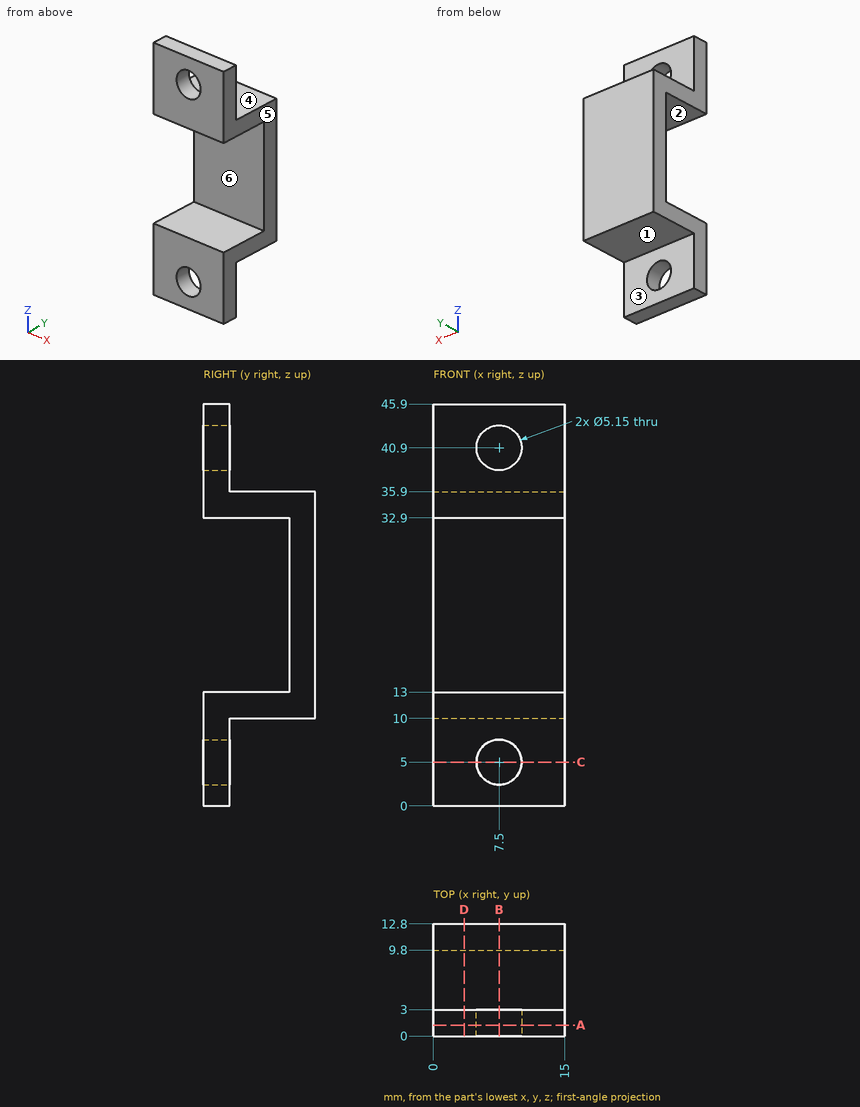
Job drawing, mm, ordinate dimensions from the low corner. One solid piece. A direction names the side the tool comes from. Round coordinates to 2 decimals unless told otherwise and drop trailing zeros. Loops run counter-clockwise (first coordinate to the right, second up) from the corner with the lowest first, then second, coordinate; pieces in that order, holes last. Notation, with made-up numbers: M -11.5,68 L 5.5,68 A34 cw 5.5,106 Z; hole C 31,83 d6. An arc over 180 degrees is marked long. One line per question, with ' | ' between items. Start each with the question number.
Item 1: Wall check: line 1 (Z direction, x = 7.5, y = 1.7) (3 decimals); line 2 (Z direction, x = 6, y = 7.5); line 3 (Z direction, x = 3.75, y = 0.5). Give the ranges that are in metal, low to high.
Item 2: Cut at C-C, the plane z = 5. Write the cut outline in (x, y) (3 decimals).
Item 3: Cut at B-B, the plane x = 7.5. Write the cut outline in (y, z) (3 decimals), plus the area to 3 significant figures.
Item 4: Cut at A-A, the plane y = 1.25. Write the cut outline in (x, z) (3 decimals), plus the area to 3 significant figures.
Item 5: Pin check, flat tips, straight feed: pin 1 Ø5 at (x, z) = (8.5, 39.5) entering from +Y; pin 2 Ø2 at (x, y) = (10.5, 9.5) entering from -Z; pin 3 Ø3 at (x, y) = (7, 6) entering from +Z. Stop position of each tip, or through.
Item 6: Cut at D-D, the plane x = 3.5. Write the cut outline in (y, z), plus the area to 4 significant figures.
Item 7: Two-plate mould, pull along Z, no slides. Class the marked faces 1, 2 and 3: pulls with the +Z half, pulls with the -Z half, needs draft (parallel to the pull), parting line crosses it, or undercut.
Item 8: Which spindle directions (+Z, -Z, +X, -X, +Y, -Y) get a long thin tool onto all of the face, cutting with end or side? Do the marked faces 4, 5 and 6. Say none if no direction does.
Responses:
1) line 1: z = 0 to 2.425, 7.575 to 13, 32.9 to 38.325, 43.475 to 45.9 | line 2: z = 10 to 13, 32.9 to 35.9 | line 3: z = 0 to 13, 32.9 to 45.9
2) outline: M 0,0 L 4.925,0 L 4.925,3 L 0,3 Z; M 10.075,0 L 15,0 L 15,3 L 10.075,3 Z
3) outline: M 0,0 L 3,0 L 3,2.425 L 0,2.425 Z; M 0,7.575 L 3,7.575 L 3,10 L 12.8,10 L 12.8,35.9 L 3,35.9 L 3,38.325 L 0,38.325 L 0,32.9 L 9.8,32.9 L 9.8,13 L 0,13 Z; M 0,43.475 L 3,43.475 L 3,45.9 L 0,45.9 Z | area: 166 mm²
4) outline: M 0,0 L 15,0 L 15,13 L 0,13 Z; M 0,32.9 L 15,32.9 L 15,45.9 L 0,45.9 Z; hole C 7.5,5 d5.15; hole C 7.5,40.9 d5.15 | area: 348 mm²
5) pin 1: stops at y = 3 | pin 2: stops at z = 10 | pin 3: stops at z = 35.9
6) outline: M 0,0 L 3,0 L 3,10 L 12.8,10 L 12.8,35.9 L 3,35.9 L 3,45.9 L 0,45.9 L 0,32.9 L 9.8,32.9 L 9.8,13 L 0,13 Z | area: 196.5 mm²
7) face 1: pulls with the -Z half | face 2: undercut | face 3: needs draft
8) face 4: +Z, +X, -X, +Y | face 5: +Z, -Z, +X, +Y, -Y | face 6: +X, -X, -Y
